CAD build for the part. Positions are in the model's coordinates, mm. Coordinates: 2 decimals unless noted, no trailing zeros. Write each loop counter-clockwise with the first axis right and the second up, starting at its lowest first coordinate (ties: lowest second). Pieces come first, ordered by that corner, then holes. Notation, with made-up numbers: (33, 58) - (47, 58) arc R22 ccw to (47, 75) - close; hole circle Ø5 at (84, 33). An arc over 180 degrees is marked (long way). Answer in a Markdown table with one row per item. Add a question column.
Q1. Drill centre lines: line 1 along X through (y, z) = (-0.7, 55); line 2 along Z through (x, y) = (-75, -1.95); line 3 along Z through (x, y) = (-60.5, -1.15). Where is each one in solid material? Low to high. Write a range as from..to.
Q2. Two-plate mould, pull along X, no slides. Class faces 1 (the flat face through (-1, -3, 41)), 2 (the cylindrical face through (-78, -1, 59)), 3 (the cylindrical face through (36.633, -1.521, 38.495)), 4 (the cylindrical face through (78, -1, -59)): +X half, -X half, draft (parallel to the pull), parting line (faces both ways), or undercut.
Q3. Band-saw the part on B-B (x = -43). List the corners of the cut face in (y, z).
Q4. Band-saw the part on A-A (z = -38.5). List the corners of the cut face in (x, y).
Q5. Band-saw the part on C-C (y = -1.05). State how many separate pieces and enclosed holes the cut face has, and give its area (3 significant figures).
Q6. Pin check, flat tip, straight feed: pin 1 (4 mm diameter, centred on x = 52.5, z = 34.4, fed in from +Y). Stop position of the tip, or through.
```python
from build123d import *

# Parameters (mm, degrees)
F1_DEPTH = 3
F2_R     = 1.5
F3_DEPTH = 25
F4_R     = 1.5
F5_DEPTH = 25
F6_W     = 121
F6_H     = 76
F6_R     = 1.5
F7_DEPTH = 3
F8_R     = 4
F9_DEPTH = 3


# Not quite as in the source:
# - a feature names something its author has since deleted; it is built from what else it names


with BuildPart() as f1:
    # F0 (on Front) → F1 (new body)
    with BuildSketch(Plane.XZ):
        with BuildLine():
            Line((-75, -60), (75, -60))
            ThreePointArc((75, -60), (78.5355339059, -58.5355339059), (80, -55))
            Line((80, -55), (80, 55))
            ThreePointArc((80, 55), (78.5355339059, 58.5355339059), (75, 60))
            Line((75, 60), (-75, 60))
            ThreePointArc((-75, 60), (-78.5355339059, 58.5355339059), (-80, 55))
            Line((-80, 55), (-80, -55))
            ThreePointArc((-80, -55), (-78.5355339059, -58.5355339059), (-75, -60))
        make_face()
    extrude(amount=F1_DEPTH)

    # F2 (on Front) → F3 (cut)
    with BuildSketch(Plane.XZ):
        with Locations((-75, 55)):
            Circle(F2_R)
        with Locations((75, 55)):
            Circle(F2_R)
        with Locations((75, -55)):
            Circle(F2_R)
        with Locations((-75, -55)):
            Circle(F2_R)
    extrude(amount=F3_DEPTH, mode=Mode.SUBTRACT)

    # F4 (on Front) → F5 (cut)
    with BuildSketch(Plane.XZ):
        with Locations((52.5, 34.4)):
            Circle(F4_R)
    extrude(amount=F5_DEPTH, mode=Mode.SUBTRACT)

    # F6 (on face) → F7 (cut)
    with BuildSketch(Plane.XZ.offset(3)):
        with Locations((-4, -7.6)):
            Rectangle(F6_W, F6_H)
        with Locations((52.5, 34.4)):
            Circle(F6_R)
        with Locations((-60.5, 34.4)):
            Circle(F6_R)
        with Locations((-60.5, -49.6)):
            Circle(F6_R)
        with Locations((52.5, -49.6)):
            Circle(F6_R)
    extrude(amount=-F7_DEPTH, mode=Mode.SUBTRACT)

    # F8 (on face) → F9 (cut)
    with BuildSketch(Plane.XZ.offset(3)):
        with Locations((37.5, 42.4)):
            Circle(F8_R)
    extrude(amount=-F9_DEPTH, mode=Mode.SUBTRACT)


solid = f1.part
```
Checked values:
| question | item | result |
|---|---|---|
| 1 | line 1 | x = -80..-76.5, -73.5..73.5, 76.5..80 |
| 1 | line 2 | z = -60..-56.5, -53.5..53.5, 56.5..60 |
| 1 | line 3 | z = -60..-51.1, -48.1..-45.6, 30.4..32.9, 35.9..60 |
| 2 | face 1 | draft |
| 2 | face 2 | -X half |
| 2 | face 3 | undercut |
| 2 | face 4 | +X half |
| 3 | outline | (-3, -60) - (0, -60) - (0, -45.6) - (-3, -45.6) - close; (-3, 30.4) - (0, 30.4) - (0, 60) - (-3, 60) - close |
| 4 | outline | (-80, -3) - (-64.5, -3) - (-64.5, 0) - (-80, 0) - close; (56.5, -3) - (80, -3) - (80, 0) - (56.5, 0) - close |
| 5 | separate pieces | 1 |
| 5 | enclosed holes | 10 |
| 5 | area | 9,880 mm² |
| 6 | pin 1 | stops at y = 0 |
